Can you work these out from the model? Positions are in its coordinate system, mm. Face numbers are marked on the shaded views. A direction names the side the tool comes from. Coordinates: 2 decimals unless noted, no trailing zeros. Order: outer loops, then holes, each group sorted by start corner. A loop starts at its lowest first (then second) coordinate and runs counter-clockwise, first axis right, second up.
```python
from build123d import *


with BuildPart() as part:
    # 草图1 → 旋转1 (revolve)
    with BuildSketch(Plane(origin=(0, 0, 0), x_dir=(1, 0, 0), z_dir=(0, 1, 0))):
        with BuildLine():
            Line((0, 31), (0, 26))
            Line((0, 26), (0, -26))
            Line((0, -26), (55, -26))
            Line((55, -26), (55, -20))
            Line((55, -20), (80, -20))
            ThreePointArc((80, -20), (83.535533906, -18.535533906), (85, -15))
            Line((85, -15), (85, 15))
            ThreePointArc((85, 15), (83.535533906, 18.535533906), (80, 20))
            Line((80, 20), (55, 20))
            Line((55, 20), (55, 26))
            Line((55, 26), (5, 26))
            Line((5, 26), (5, 31))
            Line((5, 31), (0, 31))
        make_face()
    revolve(axis=Axis((0, 0, -26), (0, 0, -1)))


solid = part.part
```
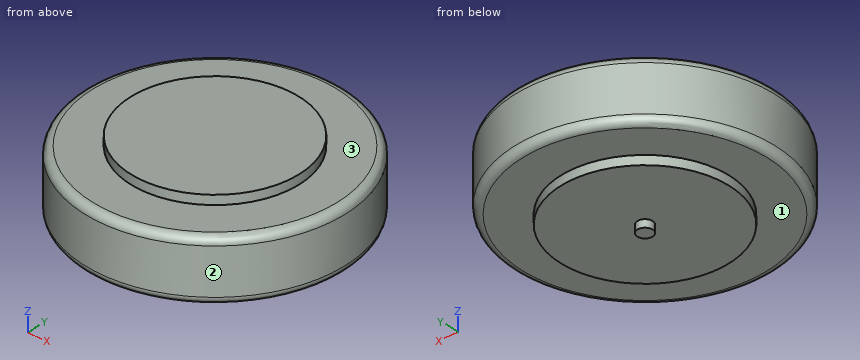
1. On a 3-axis mill with a long thin cutter (end or side, diameter ignored), from which of +Z, -Z, +X, -X, +Y, -Y can I reach the whole of each face in a straight line? I mean the marked faces 1, 2 and 3. Say none if no direction works.
Completed:
face 1: -Z
face 2: +Z, -Z
face 3: +Z
2. Imagine slicing it at A-A on x = 0. Please give me the cut outline in (y, z).
Completed:
outline: (-85, -15) arc R5 ccw to (-80, -20) - (-55, -20) - (-55, -26) - (-5, -26) - (-5, -31) - (5, -31) - (5, -26) - (55, -26) - (55, -20) - (80, -20) arc R5 ccw to (85, -15) - (85, 15) arc R5 ccw to (80, 20) - (55, 20) - (55, 26) - (-55, 26) - (-55, 20) - (-80, 20) arc R5 ccw to (-85, 15) - close
3. Please list where these lines run through material, in increasing order: probe 1 along Z at (x, y) = (13.5, -23); probe 2 along Z at (x, y) = (-61, -50); probe 3 along X at (y, z) = (20, 2).
Completed:
probe 1: z = -26 to 26
probe 2: z = -20 to 20
probe 3: x = -82.61 to 82.61
4. Imagine slicing it at C-C on z = -9. Please give me the cut outline in (x, y).
Completed:
outline: circle Ø170 at (0, 0)
5. I'm going to push flat-ended pins straight in: pin 1 (8 mm diameter, centred on x = -36.5, y = 54.5, fed in from -Z); pin 2 (10 mm diameter, centred on y = 64.5, z = 5.5, fed in from -X); pin 3 (1 mm diameter, centred on x = -54, z = 10.5, fed in from +Y). Where does each tip first touch, or does it pass through?
Completed:
pin 1: stops at z = -20
pin 2: stops at x = -60.7
pin 3: stops at y = 66.05
